Verification items for this drawing (mm, ordinates from the low corner). Round coordinates to 2 decimals unless told otherwise and drop trailing zeros. Write each loop counter-clockwise with the first axis right and the second up, starting at its lowest first coordinate (ties: lowest second). Pieces come first, ordered by that corner, then holes. Notation, with made-up numbers: M 19.5,76.5 L 59.5,76.5 A23 ccw 59.5,84.5 Z; hole C 10,1.5 d8. An arc over 180 degrees is marked long. Write each question's results on one line, items separated by ' | '.
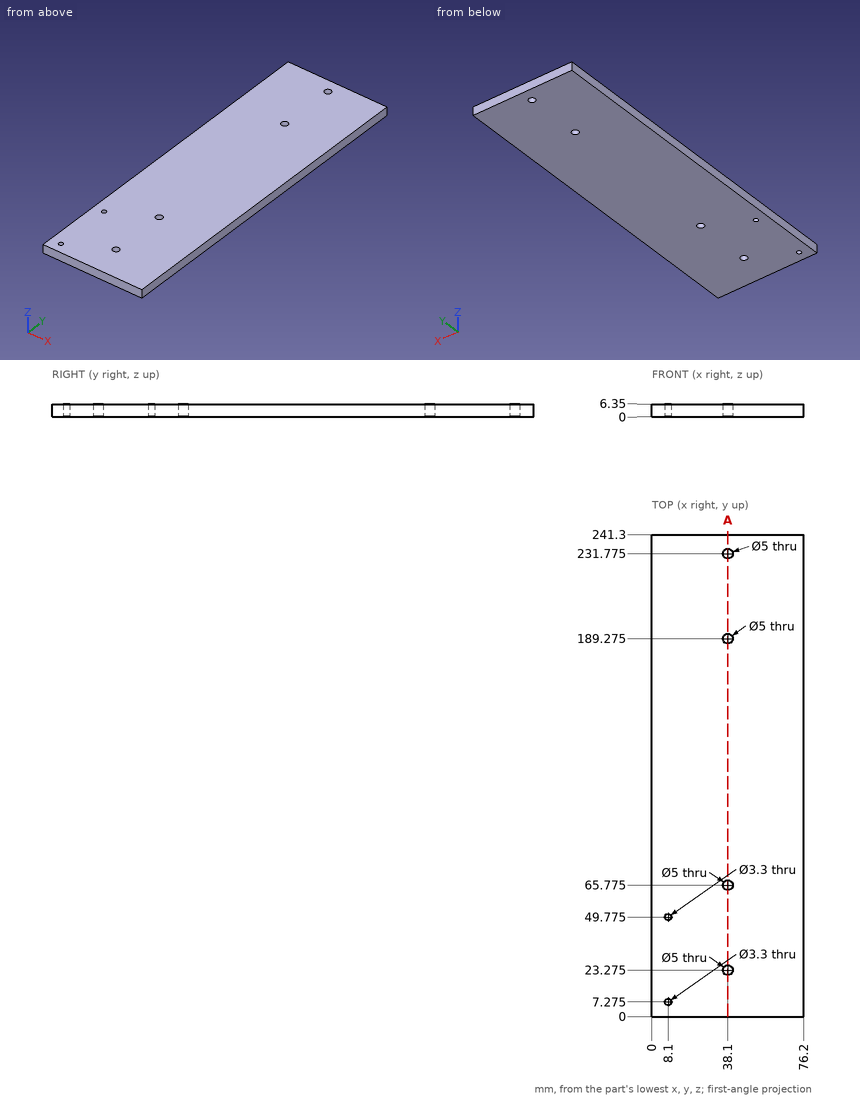
1) Sectioned sample at A-A, the plane x = 38.1. Record the cut outline in (y, z) (3 decimals).
Calculated:
outline: M 0,0 L 20.775,0 L 20.775,6.35 L 0,6.35 Z; M 25.775,0 L 63.275,0 L 63.275,6.35 L 25.775,6.35 Z; M 68.275,0 L 186.775,0 L 186.775,6.35 L 68.275,6.35 Z; M 191.775,0 L 229.275,0 L 229.275,6.35 L 191.775,6.35 Z; M 234.275,0 L 241.3,0 L 241.3,6.35 L 234.275,6.35 Z
2) Depth check by flat-ended pin: P1, Ø3, axis at x = 8.1, y = 49.775, coming from the -Z side. Enter the tip coordinate at first touch or a pass-through.
Calculated:
P1: passes through
3) Material ranges on line 1 (Y direction, x = 8.1, z = 4.5) (3 decimals); line 2 (Y direction, x = 38.1, z = 3) (3 decimals); line 3 (Y direction, x = 39, z = 6), recorded low to high. Write a range as [from, to].
Calculated:
line 1: y = [0, 5.625], [8.925, 48.125], [51.425, 241.3] | line 2: y = [0, 20.775], [25.775, 63.275], [68.275, 186.775], [191.775, 229.275], [234.275, 241.3] | line 3: y = [0, 20.94], [25.61, 63.44], [68.11, 186.94], [191.61, 229.44], [234.11, 241.3]
